The model under review builds one solid part; all positions refer to its coordinate system, in mm. Face numbers are marked on the shaded views. A direction names the side the tool comes from. Round coordinates to 2 decimals unless told otherwise and drop trailing zeros. Loops run counter-clockwise (first coordinate to the right, second up) from the corner with the lowest first, then second, coordinate; pieces in that order, holes last. Notation, with made-up numbers: (17, -10.5) -> (21, -10.5) arc R17 cw to (21, 2.5) -> close; hole circle Ø9 at (42.5, -1.5). An arc over 180 degrees is marked (long way). Use a Markdown table: item, result. Add a question column.
1) Consider section C-C on y = 34. Give the boundary of the cut face in (x, z).
2) Consider section B-B on x = 14.5. Give the boundary of the cut face in (y, z).
3) Wall thickness on probe 1 along Y at (x, z) = (22.5, 21); probe 2 along Y at (x, z) = (15.5, 14.25); probe 3 along Y at (x, z) = (-15, 4.5): over which ranges is each line inside the solid? List them lowest first.
4) Insertion check: pin 1 (1.5 mm diameter, centred on y = 70, z = 7.5, fed in from +X); pin 2 (9.5 mm diameter, centred on x = -19, z = 6.5, fed in from +Y) (3 decimals); pin 3 (7 mm diameter, centred on x = 13.5, z = 11, fed in from +Y). Each pin has a flat end and moves straight along its axis. Give the tip position at first contact, or say it passes through.
5) Consider section A-A on z = 16.25. Give the boundary of the cut face in (x, y), plus the area to 3 significant figures.
6) Mouldability with a two-part tool opening along X and no side actions: class the marked faces 5, 6 and 7 as released by +X, released by -X, zero draft, split by the parting line, or undercut.
7) For the marked faces 1, 2, 3 and 4, list the 3-axis set-ups (+Z, -Z, +X, -X, +Y, -Y) from which the entire face can be reached by the end or side of a thin tool; tool diameter is ignored.
8) Consider section D-D on x = 34. Give the boundary of the cut face in (y, z).
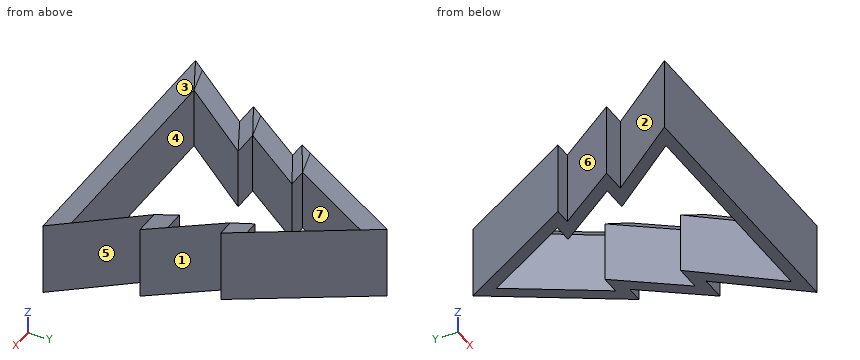
from build123d import *

# Parameters (mm, degrees)
F1_DEPTH     = 25.4
F2_T4_DEPTH  = 57.8731292872
F2_T9_DEPTH  = 41.0926802964
F2_T14_DEPTH = 63.860720941
F2_T19_DEPTH = 105.3637727113
F2_T25_DEPTH = 63.860720941
F2_T30_DEPTH = 41.0926802964
F2_T35_DEPTH = 57.8731292872
F2_T40_DEPTH = 38.84406527
F2_T45_DEPTH = 65.6766537471
F2_T51_DEPTH = 65.6766537471
F2_T57_DEPTH = 38.84406527


# Not quite as in the source:
# - a fillet or chamfer that OpenCascade refuses, or shapes differently, is made with other operations: its cross-section is extruded or revolved along the edge and cut away or added


with BuildPart() as f1:
    # F0 (on Top) → F1 (new body)
    with BuildSketch(Plane.XY):
        Polygon((-44.2180235174, 0.5666213692), (0, 0.5666213692), (44.2180235174, 0.5666213692), (24.8746419192, 25.0471287349), (32.8946120205, 25.0471287349), (18.1270946377, 45.4824770849), (23.5501605907, 45.4824770849), (0, 85.1436531389), (-23.5501605907, 45.4824770849), (-18.1270946377, 45.4824770849), (-32.8946120205, 25.0471287349), (-24.8746419192, 25.0471287349), align=None)
        Polygon((36.3516993821, 4.3766213692), (0, 4.3766213692), (-36.3516993821, 4.3766213692), (-17.0083177839, 28.8571287349), (-25.4406241332, 28.8571287349), (-10.6731067504, 49.2924770849), (-16.8567980732, 49.2924770849), (0, 77.6812616757), (16.8567980732, 49.2924770849), (10.6731067504, 49.2924770849), (25.4406241332, 28.8571287349), (17.0083177839, 28.8571287349), align=None, mode=Mode.SUBTRACT)
    extrude(amount=F1_DEPTH)

    # F2: chamfer of 6.35 on 11 edges, made by hand


with BuildPart() as f2_tool2:
    # F2_s3 → F2_t4 (new body)
    with BuildSketch(Plane(origin=(-29.3040400955, 40.5510453716, 0), x_dir=(0, 0, 1), z_dir=(0.585716126, -0.8105162674, 0))):
        Polygon((25.4, -43.8721253629), (19.05, -37.5221253629), (25.4, -37.5221253629), align=None)
    extrude(amount=F2_T4_DEPTH)

    split(bisect_by=Plane(origin=(0, 23.9535643674, 23.9535643674), x_dir=(1, 0, 0), z_dir=(0, 0.7071067812, 0.7071067812)), keep=Keep.TOP)


with BuildPart() as f1_1:
    add(f1.part)

    # F2_t1: cut F2_tool2
    add(f2_tool2.part, mode=Mode.SUBTRACT)


with BuildPart() as f2_tool7:
    # F2_s8 → F2_t9 (new body)
    with BuildSketch(Plane.YZ.offset(41.7708111067)):
        Polygon((22.5071287349, 25.4), (28.8571287349, 19.05), (28.8571287349, 25.4), align=None)
    extrude(amount=-F2_T9_DEPTH)

    split(bisect_by=Plane(origin=(7.4859790504, 5.409710853, -9.2360626814), x_dir=(0.585716126, -0.8105162674, 0), z_dir=(-0.573121549, -0.4141638445, 0.7071067812)), keep=Keep.TOP)


with BuildPart() as f1_2:
    add(f1_1.part)

    # F2_t6: cut F2_tool7
    add(f2_tool7.part, mode=Mode.SUBTRACT)


with BuildPart() as f2_tool12:
    # F2_s13 → F2_t14 (new body)
    with BuildSketch(Plane(origin=(-17.6242588903, 22.3048280047, 0), x_dir=(0, 0, 1), z_dir=(0.6199732843, -0.7846229201, 0))):
        Polygon((25.4, -37.5857648435), (19.05, -31.2357648435), (25.4, -31.2357648435), align=None)
    extrude(amount=F2_T14_DEPTH)

    split(bisect_by=Plane(origin=(0, 11.7133106846, 11.7133106846), x_dir=(1, 0, 0), z_dir=(0, 0.7071067812, 0.7071067812)), keep=Keep.TOP)


with BuildPart() as f1_3:
    add(f1_2.part)

    # F2_t11: cut F2_tool12
    add(f2_tool12.part, mode=Mode.SUBTRACT)


with BuildPart() as f2_tool17:
    # F2_s18 → F2_t19 (new body)
    with BuildSketch(Plane.YZ.offset(-52.6818863557)):
        Polygon((-1.9733786308, 25.4), (4.3766213692, 19.05), (4.3766213692, 25.4), align=None)
    extrude(amount=F2_T19_DEPTH)

    split(bisect_by=Plane(origin=(4.7806151974, 3.7774243261, -6.0928824217), x_dir=(0.6199732843, -0.7846229201, 0), z_dir=(-0.5548121875, -0.4383873135, 0.7071067812)), keep=Keep.TOP)

    split(bisect_by=Plane(origin=(-4.7806151974, 3.7774243261, -6.0928824217), x_dir=(0.6199732843, 0.7846229201, 0), z_dir=(0.5548121875, -0.4383873135, 0.7071067812)), keep=Keep.TOP)


with BuildPart() as f1_4:
    add(f1_3.part)

    # F2_t16: cut F2_tool17
    add(f2_tool17.part, mode=Mode.SUBTRACT)


with BuildPart() as f2_tool23:
    # F2_s24 → F2_t25 (new body)
    with BuildSketch(Plane(origin=(-21.9676820116, -27.8017573382, 0), x_dir=(0, 0, 1), z_dir=(0.6199732843, 0.7846229201, 0))):
        Polygon((25.4, -37.5857648435), (19.05, -31.2357648435), (25.4, -31.2357648435), align=None)
    extrude(amount=F2_T25_DEPTH)

    split(bisect_by=Plane(origin=(0, 11.7133106846, 11.7133106846), x_dir=(1, 0, 0), z_dir=(0, 0.7071067812, 0.7071067812)), keep=Keep.TOP)


with BuildPart() as f1_5:
    add(f1_4.part)

    # F2_t22: cut F2_tool23
    add(f2_tool23.part, mode=Mode.SUBTRACT)


with BuildPart() as f2_tool28:
    # F2_s29 → F2_t30 (new body)
    with BuildSketch(Plane.YZ.offset(-0.6781308103)):
        Polygon((22.5071287349, 25.4), (28.8571287349, 19.05), (28.8571287349, 25.4), align=None)
    extrude(amount=-F2_T30_DEPTH)

    split(bisect_by=Plane(origin=(-7.4859790504, 5.409710853, -9.2360626814), x_dir=(0.585716126, 0.8105162674, 0), z_dir=(0.573121549, -0.4141638445, 0.7071067812)), keep=Keep.TOP)


with BuildPart() as f1_6:
    add(f1_5.part)

    # F2_t27: cut F2_tool28
    add(f2_tool28.part, mode=Mode.SUBTRACT)


with BuildPart() as f2_tool33:
    # F2_s34 → F2_t35 (new body)
    with BuildSketch(Plane(origin=(-4.5931849883, -6.3560673631, 0), x_dir=(0, 0, 1), z_dir=(0.585716126, 0.8105162674, 0))):
        Polygon((25.4, -43.8721253629), (19.05, -37.5221253629), (25.4, -37.5221253629), align=None)
    extrude(amount=F2_T35_DEPTH)

    split(bisect_by=Plane(origin=(0, 23.9535643674, 23.9535643674), x_dir=(1, 0, 0), z_dir=(0, 0.7071067812, 0.7071067812)), keep=Keep.TOP)


with BuildPart() as f1_7:
    add(f1_6.part)

    # F2_t32: cut F2_tool33
    add(f2_tool33.part, mode=Mode.SUBTRACT)


with BuildPart() as f2_tool38:
    # F2_s39 → F2_t40 (new body)
    with BuildSketch(Plane.YZ.offset(5.6570802232)):
        Polygon((42.9424770849, 25.4), (49.2924770849, 19.05), (49.2924770849, 25.4), align=None)
    extrude(amount=-F2_T40_DEPTH)

    split(bisect_by=Plane(origin=(-8.8610845664, 5.2615677423, -10.3054798432), x_dir=(0.5105601896, 0.8598420162, 0), z_dir=(0.6080001204, -0.3610205722, 0.7071067812)), keep=Keep.TOP)


with BuildPart() as f1_8:
    add(f1_7.part)

    # F2_t37: cut F2_tool38
    add(f2_tool38.part, mode=Mode.SUBTRACT)


with BuildPart() as f2_tool43:
    # F2_s44 → F2_t45 (new body)
    with BuildSketch(Plane(origin=(8.9078181115, 15.0017890968, 0), x_dir=(0, 0, 1), z_dir=(0.5105601896, 0.8598420162, 0))):
        Polygon((25.4, -46.0109596864), (19.05, -39.6609596864), (25.4, -39.6609596864), align=None)
    extrude(amount=F2_T45_DEPTH)

    split(bisect_by=Plane(origin=(0, 34.1712385424, 34.1712385424), x_dir=(1, 0, 0), z_dir=(0, 0.7071067812, 0.7071067812)), keep=Keep.TOP)

    split(bisect_by=Plane(origin=(8.8610845664, 5.2615677423, -10.3054798432), x_dir=(0.5105601896, -0.8598420162, 0), z_dir=(-0.6080001204, -0.3610205722, 0.7071067812)), keep=Keep.TOP)


with BuildPart() as f1_9:
    add(f1_8.part)

    # F2_t42: cut F2_tool43
    add(f2_tool43.part, mode=Mode.SUBTRACT)


with BuildPart() as f2_tool49:
    # F2_s50 → F2_t51 (new body)
    with BuildSketch(Plane(origin=(-42.4397028983, 71.4733354725, 0), x_dir=(0, 0, 1), z_dir=(0.5105601896, -0.8598420162, 0))):
        Polygon((25.4, -46.0109596864), (19.05, -39.6609596864), (25.4, -39.6609596864), align=None)
    extrude(amount=F2_T51_DEPTH)

    split(bisect_by=Plane(origin=(-8.8610845664, 5.2615677423, -10.3054798432), x_dir=(0.5105601896, 0.8598420162, 0), z_dir=(0.6080001204, -0.3610205722, 0.7071067812)), keep=Keep.TOP)

    split(bisect_by=Plane(origin=(0, 34.1712385424, 34.1712385424), x_dir=(1, 0, 0), z_dir=(0, 0.7071067812, 0.7071067812)), keep=Keep.TOP)


with BuildPart() as f1_10:
    add(f1_9.part)

    # F2_t48: cut F2_tool49
    add(f2_tool49.part, mode=Mode.SUBTRACT)


with BuildPart() as f2_tool55:
    # F2_s56 → F2_t57 (new body)
    with BuildSketch(Plane.YZ.offset(33.1869850468)):
        Polygon((42.9424770849, 25.4), (49.2924770849, 19.05), (49.2924770849, 25.4), align=None)
    extrude(amount=-F2_T57_DEPTH)

    split(bisect_by=Plane(origin=(8.8610845664, 5.2615677423, -10.3054798432), x_dir=(0.5105601896, -0.8598420162, 0), z_dir=(-0.6080001204, -0.3610205722, 0.7071067812)), keep=Keep.TOP)


with BuildPart() as f1_11:
    add(f1_10.part)

    # F2_t54: cut F2_tool55
    add(f2_tool55.part, mode=Mode.SUBTRACT)


solid = f1_11.part
Result set:
| question | item | result |
|---|---|---|
| 1 | outline | (-26.42, 0) -> (-21.72, 0) -> (-21.72, 19.05) -> (-26.42, 22.86) -> close; (21.72, 0) -> (26.42, 0) -> (26.42, 22.86) -> (21.72, 19.05) -> close |
| 2 | outline | (0.57, 0) -> (4.38, 0) -> (4.38, 19.05) -> (0.57, 22.86) -> close; (44, 0) -> (49.29, 0) -> (49.29, 19.05) -> (47.34, 21.01) -> (44, 19.05) -> close; (53.26, 0) -> (60.72, 0) -> (60.72, 22.86) -> (53.26, 19.05) -> close |
| 3 | probe 1 | 0.57 to 2.43, 25.05 to 26.91, 36.26 to 39.43, 45.48 to 47.25 |
| 3 | probe 2 | 0.57 to 4.38, 42.61 to 49.29, 51.58 to 59.04 |
| 3 | probe 3 | 0.57 to 4.38, 43.3 to 49.29, 52.42 to 59.88 |
| 4 | pin 1 | x = 9.44 |
| 4 | pin 2 | y = 61.145 |
| 4 | pin 3 | y = 68.3 |
| 5 | outline | (-44.22, 0.57) -> (44.22, 0.57) -> (24.87, 25.05) -> (32.89, 25.05) -> (18.13, 45.48) -> (23.55, 45.48) -> (0, 85.14) -> (-23.55, 45.48) -> (-18.13, 45.48) -> (-32.89, 25.05) -> (-24.87, 25.05) -> close; hole (-36.35, 4.38) -> (36.35, 4.38) -> (17.01, 28.86) -> (25.44, 28.86) -> (10.67, 49.29) -> (16.86, 49.29) -> (0, 77.68) -> (-16.86, 49.29) -> (-10.67, 49.29) -> (-25.44, 28.86) -> (-17.01, 28.86) -> close |
| 5 | area | 1,150 mm2 |
| 6 | face 5 | released by +X |
| 6 | face 6 | released by -X |
| 6 | face 7 | undercut |
| 7 | face 1 | +Z, -Z, +X |
| 7 | face 2 | +Z, -Z, -X |
| 7 | face 3 | +Z |
| 7 | face 4 | +Z, -Z |
| 8 | outline | (0.57, 0) -> (4.38, 0) -> (4.38, 19.05) -> (0.57, 22.86) -> close; (7.35, 0) -> (13.5, 0) -> (13.5, 22.86) -> (7.35, 19.05) -> close |
